```python
from build123d import *

# Parameters (mm, degrees)
F1_DEPTH = 8
F3_DEPTH = 2
F5_D     = 3.5
F5_DEPTH = 8
F5_TIP   = 1.0515060833


with BuildPart() as f1:
    # F0 (on Top) → F1 (new body)
    with BuildSketch(Plane.XY):
        Polygon((20, -8.2842712475), (20, 8.2842712475), (8.2842712475, 20), (-8.2842712475, 20), (-20, 8.2842712475), (-20, -8.2842712475), (-8.2842712475, -20), (8.2842712475, -20), align=None)
    extrude(amount=F1_DEPTH)

    # F2 (on face) → F3 (cut)
    with BuildSketch(Plane.XY.offset(8)):
        Polygon((18, -7.4558441227), (18, 7.4558441227), (7.4558441227, 18), (-7.4558441227, 18), (-18, 7.4558441227), (-18, -7.4558441227), (-7.4558441227, -18), (7.4558441227, -18), align=None)
        with BuildLine():
            add(Edge.make_bspline(
                [(-11.0686569032, -0.7610464389), (-10.4772186757, -1.4050569533), (-10.4772186757, -2.4302165478)],
                knots=[0, 0, 0, 1, 1, 1], degree=2))
            add(Edge.make_bspline(
                [(-10.4772186757, -2.4302165478), (-10.4772186757, -3.751095256), (-11.4355676555, -4.4914882964)],
                knots=[0, 0, 0, 1, 1, 1], degree=2))
            add(Edge.make_bspline(
                [(-11.4355676555, -4.4914882964), (-12.3939166354, -5.2318813368), (-14.0368006008, -5.2318813368)],
                knots=[0, 0, 0, 1, 1, 1], degree=2))
            add(Edge.make_bspline(
                [(-14.0368006008, -5.2318813368), (-15.8154963074, -5.2318813368), (-16.7749405432, -4.7718738265)],
                knots=[0, 0, 0, 1, 1, 1], degree=2))
            Line((-16.7749405432, -4.7718738265), (-16.7749405432, -3.6503317061))
            add(Edge.make_bspline(
                [(-16.7749405432, -3.6503317061), (-16.1572161722, -3.9088121167), (-15.4321567155, -4.0599574415)],
                knots=[0, 0, 0, 1, 1, 1], degree=2))
            add(Edge.make_bspline(
                [(-15.4321567155, -4.0599574415), (-14.7070972587, -4.2111027663), (-13.9951808737, -4.2111027663)],
                knots=[0, 0, 0, 1, 1, 1], degree=2))
            add(Edge.make_bspline(
                [(-13.9951808737, -4.2111027663), (-12.8320190262, -4.2111027663), (-12.2427713106, -3.7697146076)],
                knots=[0, 0, 0, 1, 1, 1], degree=2))
            add(Edge.make_bspline(
                [(-12.2427713106, -3.7697146076), (-11.6535235949, -3.3283264489), (-11.6535235949, -2.5397421454)],
                knots=[0, 0, 0, 1, 1, 1], degree=2))
            add(Edge.make_bspline(
                [(-11.6535235949, -2.5397421454), (-11.6535235949, -2.0205908124), (-11.8627174865, -1.6887282513)],
                knots=[0, 0, 0, 1, 1, 1], degree=2))
            add(Edge.make_bspline(
                [(-11.8627174865, -1.6887282513), (-12.0719113781, -1.3568656903), (-12.5614907998, -1.0753849042)],
                knots=[0, 0, 0, 1, 1, 1], degree=2))
            add(Edge.make_bspline(
                [(-12.5614907998, -1.0753849042), (-13.0510702216, -0.7939041182), (-14.0499436725, -0.4390411816)],
                knots=[0, 0, 0, 1, 1, 1], degree=2))
            add(Edge.make_bspline(
                [(-14.0499436725, -0.4390411816), (-15.4452997872, 0.0603955439), (-16.0444048066, 0.7449305295)],
                knots=[0, 0, 0, 1, 1, 1], degree=2))
            add(Edge.make_bspline(
                [(-16.0444048066, 0.7449305295), (-16.643509826, 1.4294655151), (-16.643509826, 2.5312930279)],
                knots=[0, 0, 0, 1, 1, 1], degree=2))
            add(Edge.make_bspline(
                [(-16.643509826, 2.5312930279), (-16.643509826, 3.6878833396), (-15.7749718363, 4.3724183252)],
                knots=[0, 0, 0, 1, 1, 1], degree=2))
            add(Edge.make_bspline(
                [(-15.7749718363, 4.3724183252), (-14.9064338465, 5.0569533108), (-13.4738390287, 5.0569533108)],
                knots=[0, 0, 0, 1, 1, 1], degree=2))
            add(Edge.make_bspline(
                [(-13.4738390287, 5.0569533108), (-11.982100388, 5.0569533108), (-10.7291275504, 4.5093253223)],
                knots=[0, 0, 0, 1, 1, 1], degree=2))
            Line((-10.7291275504, 4.5093253223), (-11.0927525347, 3.4973087996))
            add(Edge.make_bspline(
                [(-11.0927525347, 3.4973087996), (-12.3325823007, 4.0164601327), (-13.5023156841, 4.0164601327)],
                knots=[0, 0, 0, 1, 1, 1], degree=2))
            add(Edge.make_bspline(
                [(-13.5023156841, 4.0164601327), (-14.4267117286, 4.0164601327), (-14.9469583177, 3.619977469)],
                knots=[0, 0, 0, 1, 1, 1], degree=2))
            add(Edge.make_bspline(
                [(-14.9469583177, 3.619977469), (-15.4672049067, 3.2234948054), (-15.4672049067, 2.5181499562)],
                knots=[0, 0, 0, 1, 1, 1], degree=2))
            add(Edge.make_bspline(
                [(-15.4672049067, 2.5181499562), (-15.4672049067, 1.9989986231), (-15.2755351108, 1.6660408061)],
                knots=[0, 0, 0, 1, 1, 1], degree=2))
            add(Edge.make_bspline(
                [(-15.2755351108, 1.6660408061), (-15.0838653148, 1.3330829891), (-14.6282388284, 1.0559832269)],
                knots=[0, 0, 0, 1, 1, 1], degree=2))
            add(Edge.make_bspline(
                [(-14.6282388284, 1.0559832269), (-14.172612342, 0.7788834648), (-13.2350732257, 0.4437351358)],
                knots=[0, 0, 0, 1, 1, 1], degree=2))
            add(Edge.make_bspline(
                [(-13.2350732257, 0.4437351358), (-11.6600951308, -0.1170359244), (-11.0686569032, -0.7610464389)],
                knots=[0, 0, 0, 1, 1, 1], degree=2))
        make_face(mode=Mode.SUBTRACT)
        Polygon((-5.3492301915, 3.8806483915), (-5.3492301915, -5.0938790837), (-6.5123920391, -5.0938790837), (-6.5123920391, 3.8806483915), (-9.6820628364, 3.8806483915), (-9.6820628364, 4.9145700338), (-2.1795593942, 4.9145700338), (-2.1795593942, 3.8806483915), align=None, mode=Mode.SUBTRACT)
        with BuildLine():
            add(Edge.make_bspline(
                [(6.8037301289, 3.7032169233), (8.0150832395, 2.3341469521), (8.0150832395, -0.0754161973)],
                knots=[0, 0, 0, 1, 1, 1], degree=2))
            add(Edge.make_bspline(
                [(8.0150832395, -0.0754161973), (8.0150832395, -2.4784078107), (6.799349105, -3.8551445738)],
                knots=[0, 0, 0, 1, 1, 1], degree=2))
            add(Edge.make_bspline(
                [(6.799349105, -3.8551445738), (5.5836149706, -5.2318813368), (3.421579672, -5.2318813368)],
                knots=[0, 0, 0, 1, 1, 1], degree=2))
            add(Edge.make_bspline(
                [(3.421579672, -5.2318813368), (1.2113531105, -5.2318813368), (0.0098573038, -3.8792402053)],
                knots=[0, 0, 0, 1, 1, 1], degree=2))
            add(Edge.make_bspline(
                [(0.0098573038, -3.8792402053), (-1.1916385029, -2.5265990737), (-1.1916385029, -0.0622731255)],
                knots=[0, 0, 0, 1, 1, 1], degree=2))
            add(Edge.make_bspline(
                [(-1.1916385029, -0.0622731255), (-1.1916385029, 2.382338215), (0.0131430717, 3.7273125548)],
                knots=[0, 0, 0, 1, 1, 1], degree=2))
            add(Edge.make_bspline(
                [(0.0131430717, 3.7273125548), (1.2179246464, 5.0722868945), (3.4347227438, 5.0722868945)],
                knots=[0, 0, 0, 1, 1, 1], degree=2))
            add(Edge.make_bspline(
                [(3.4347227438, 5.0722868945), (5.5923770184, 5.0722868945), (6.8037301289, 3.7032169233)],
                knots=[0, 0, 0, 1, 1, 1], degree=2))
        make_face(mode=Mode.SUBTRACT)
        with BuildLine():
            add(Edge.make_bspline(
                [(12.840781074, 4.9145700338), (16.5909375391, 4.9145700338), (16.5909375391, 1.9989986231)],
                knots=[0, 0, 0, 1, 1, 1], degree=2))
            add(Edge.make_bspline(
                [(16.5909375391, 1.9989986231), (16.5909375391, 0.4787833271), (15.5537301289, -0.3393728877)],
                knots=[0, 0, 0, 1, 1, 1], degree=2))
            add(Edge.make_bspline(
                [(15.5537301289, -0.3393728877), (14.5165227187, -1.1575291025), (12.5866816873, -1.1575291025)],
                knots=[0, 0, 0, 1, 1, 1], degree=2))
            Line((12.5866816873, -1.1575291025), (11.4081862561, -1.1575291025))
            Line((11.4081862561, -1.1575291025), (11.4081862561, -5.0938790837))
            Line((11.4081862561, -5.0938790837), (10.2450244086, -5.0938790837))
            Line((10.2450244086, -5.0938790837), (10.2450244086, 4.9145700338))
            Line((10.2450244086, 4.9145700338), (12.840781074, 4.9145700338))
        make_face(mode=Mode.SUBTRACT)
        with BuildLine():
            add(Edge.make_bspline(
                [(0.905776693, 2.9803479785), (0.0394292152, 1.9289022406), (0.0394292152, -0.0754161973)],
                knots=[0, 0, 0, 1, 1, 1], degree=2))
            add(Edge.make_bspline(
                [(0.0394292152, -0.0754161973), (0.0394292152, -2.1082112905), (0.905776693, -3.1596570284)],
                knots=[0, 0, 0, 1, 1, 1], degree=2))
            add(Edge.make_bspline(
                [(0.905776693, -3.1596570284), (1.7721241707, -4.2111027663), (3.421579672, -4.2111027663)],
                knots=[0, 0, 0, 1, 1, 1], degree=2))
            add(Edge.make_bspline(
                [(3.421579672, -4.2111027663), (5.0841782451, -4.2111027663), (5.9330016272, -3.1640380523)],
                knots=[0, 0, 0, 1, 1, 1], degree=2))
            add(Edge.make_bspline(
                [(5.9330016272, -3.1640380523), (6.7818250094, -2.1169733383), (6.7818250094, -0.0754161973)],
                knots=[0, 0, 0, 1, 1, 1], degree=2))
            add(Edge.make_bspline(
                [(6.7818250094, -0.0754161973), (6.7818250094, 1.9442358243), (5.9362873952, 2.9880147703)],
                knots=[0, 0, 0, 1, 1, 1], degree=2))
            add(Edge.make_bspline(
                [(5.9362873952, 2.9880147703), (5.0907497809, 4.0317937164), (3.4347227438, 4.0317937164)],
                knots=[0, 0, 0, 1, 1, 1], degree=2))
            add(Edge.make_bspline(
                [(3.4347227438, 4.0317937164), (1.7721241707, 4.0317937164), (0.905776693, 2.9803479785)],
                knots=[0, 0, 0, 1, 1, 1], degree=2))
        make_face()
        with BuildLine():
            Line((11.4081862561, 3.906934535), (11.4081862561, -0.1586556515))
            Line((11.4081862561, -0.1586556515), (12.457441482, -0.1586556515))
            add(Edge.make_bspline(
                [(12.457441482, -0.1586556515), (14.0039429215, -0.1586556515), (14.695049443, 0.340781074)],
                knots=[0, 0, 0, 1, 1, 1], degree=2))
            add(Edge.make_bspline(
                [(14.695049443, 0.340781074), (15.3861559645, 0.8402177995), (15.3861559645, 1.9442358243)],
                knots=[0, 0, 0, 1, 1, 1], degree=2))
            add(Edge.make_bspline(
                [(15.3861559645, 1.9442358243), (15.3861559645, 2.9365377394), (14.7355739141, 3.4217361372)],
                knots=[0, 0, 0, 1, 1, 1], degree=2))
            add(Edge.make_bspline(
                [(14.7355739141, 3.4217361372), (14.0849918638, 3.906934535), (12.7093503567, 3.906934535)],
                knots=[0, 0, 0, 1, 1, 1], degree=2))
            Line((12.7093503567, 3.906934535), (11.4081862561, 3.906934535))
        make_face()
    extrude(amount=-F3_DEPTH, mode=Mode.SUBTRACT)

    # F5
    with Locations(Plane.XZ.offset(20)):
        with Locations((-4, 4), (4, 4)):
            Hole(F5_D / 2, depth=F5_DEPTH)
            with Locations((0, 0, -(F5_DEPTH + F5_TIP / 2))):  # 118° drill point
                Cone(0, F5_D / 2, F5_TIP, mode=Mode.SUBTRACT)


solid = f1.part
```
Part model, mm, in its own coordinate system. A direction names the side the tool comes from. Round coordinates to 2 decimals unless told otherwise and drop trailing zeros. Loops run counter-clockwise (first coordinate to the right, second up) from the corner with the lowest first, then second, coordinate; pieces in that order, holes last.
1. 3-axis set-ups, long thin cutter, end or side, ignore diameter. For faces 1 (the face through (-9.682, 4.4, 7)), 2 (the face through (0, -20, 4)): which of +Z, -Z, +X, -X, +Y, -Y reach the whole face in a straight line?
Solutions:
face 1: +Z
face 2: +Z, -Z, +X, -X, -Y
2. Slice it at D-D (x = 12). Give the cut face in (y, z), and give its area (3 significant figures).
Solutions:
outline: (-16.28, 0) - (16.28, 0) - (16.28, 8) - (13.46, 8) - (13.46, 6) - (4.91, 6) - (4.91, 8) - (3.91, 8) - (3.91, 6) - (-0.16, 6) - (-0.16, 8) - (-1.16, 8) - (-1.16, 6) - (-13.46, 6) - (-13.46, 8) - (-16.28, 8) - close
area: 211 mm2
3. Two-plate mould, pull along X, no slides. Class faces 3 (the face through (12, 3.907, 7)), 4 (the face through (0, 0, 0)): pulls with the +X half, pulls with the -X half, needs draft (parallel to the pull), parting line crosses it, or undercut.
Solutions:
face 3: undercut
face 4: needs draft
4. Slice it at C-C (z = 1.75). Give the cut face in (x, y).
Solutions:
outline: (-20, -8.28) - (-8.28, -20) - (8.28, -20) - (20, -8.28) - (20, 8.28) - (8.28, 20) - (-8.28, 20) - (-20, 8.28) - close
5. Drill centre lines: line 1 along Y through (x, z) = (-4.5, 6.5); line 2 along Z through (x, y) = (4, -15); line 3 along X through (y, z) = (-17.25, 4). Where is each one in solid material? Low to high.
Solutions:
line 1: y = -20 to -18, 3.88 to 4.91, 18 to 20
line 2: z = 0 to 2.25, 5.75 to 6
line 3: x = -11.03 to -5.75, -2.25 to 2.25, 5.75 to 11.03
6. Slice it at B-B (y = -17). Give the cut face in (x, z).
Solutions:
outline: (-11.28, 0) - (11.28, 0) - (11.28, 8) - (8.46, 8) - (8.46, 6) - (-8.46, 6) - (-8.46, 8) - (-11.28, 8) - close; hole circle Ø3.5 at (-4, 4); hole circle Ø3.5 at (4, 4)
7. Slice it at A-A (z = 7). Count the separate pieces of the cut face and the enclosed holes in it, and give its area (3 significant figures).
Solutions:
separate pieces: 5
enclosed holes: 3
area: 350 mm2
8. Flat gauge pins, fed straight in: pin 1 (1.2 mm diameter, centred on x = 14, y = 1.5, fed in from +Z); pin 2 (1.2 mm diameter, centred on x = 12, z = 7, fed in from +Y); pin 3 (1.6 mm diameter, centred on x = 12, z = 7, fed in from +Y); pin 4 (5.5 mm diameter, centred on x = 2, y = 1.5, fed in from +Z). Where does each tip first touch, or does it go through?
Solutions:
pin 1: stops at z = 6
pin 2: stops at y = 16.88
pin 3: stops at y = 17.08
pin 4: stops at z = 8
